Input: part model. Units: mm. Frame: model coordinates. Face numbers are marked on the shaded views. A direction names the side the tool comes from. Coordinates: 2 decimals unless noted, no trailing zeros. Loops run counter-clockwise (first coordinate to the right, second up) from the corner with the lowest first, then second, coordinate; pieces in that order, holes last. Notation, with made-up numbers: M -24,51 L 3,51 A24 cw 3,79 Z; hole C -26.5,7 d10. An arc over 180 degrees is marked long. Use a Markdown table: item, result. Add a question column.
1. Section A-A on z = -8.5. Output: boundary loops of the cut face in (x, y), then the cut area to 3 significant figures.
2. Pin query (flat end, axial travel): pin 1 (5 mm diameter, centred on x = 27, z = -25.5, fed in from -Y); pin 2 (4 mm diameter, centred on x = 39.5, z = -31.5, fed in from -Y); pin 3 (2.5 mm diameter, centred on x = 46.5, z = -15, fed in from -Y); pin 4 (4 mm diameter, centred on x = 30, y = -5, fed in from +Z) (1 decimal). Return the tip coordinate at first contact, or that it passes through.
3. Section C-C on z = -15. Output: boundary loops of the cut face in (x, y).
4. Draft query along Z for the marked faces 4, 5 and 6. Return one class per face: +Z half, -Z half, draft (parallel to the pull), parting line (faces both ways), or undercut.
5. Set-up query: the marked faces 1, 2 and 3. Return all of +Z, -Z, +X, -X, +Y, -Y with unobstructed straight access to the full face (end or side cutting, diameter ignored); none if empty.
6. Section D-D on x = 41. Output: boundary loops of the cut face in (y, z), then the cut area to 3 significant figures.
7. Line query: L1, parallel to Z at x = 19, y = 6.4; L2, parallel to X at y = 5.3, z = -32; L3, parallel to Y at x = 30, z = -23. Output: solid intervals per line, ascending. Write a range as [from, to].
```python
from build123d import *
from build123d.topology import SkipClean

# Parameters (mm, degrees)
SKETCH1_W            = 60
SKETCH1_H            = 42
BOSS_EXTRUDE1_DEPTH  = 8
SKETCH3_W            = 10
SKETCH3_H            = 42
BOSS_EXTRUDE5_DEPTH  = 6
SKETCH5_W            = 14
SKETCH5_H            = 42
BOSS_EXTRUDE6_DEPTH  = 11
SKETCH6_R            = 3.2
CUT_EXTRUDE1_DEPTH   = 75.565407529
FILLET1_R            = 7
FILLET2_R            = 5
FILLET3_R            = 5
BOSS_EXTRUDE7_DEPTH  = 42
SKETCH9_W            = 5
SKETCH9_H            = 42
BOSS_EXTRUDE8_DEPTH  = 6
SKETCH11_W           = 15
SKETCH11_H           = 42
CUT_EXTRUDE2_DEPTH   = 76.921011584
SKETCH12_W           = 30
SKETCH12_H           = 42
CUT_EXTRUDE3_DEPTH   = 6
SKETCH15_W           = 42
SKETCH15_H           = 8
BOSS_EXTRUDE9_DEPTH  = 5
SKETCH16_W           = 42
SKETCH16_H           = 8
BOSS_EXTRUDE10_DEPTH = 5
CUT_EXTRUDE7_START   = -17
CUT_EXTRUDE7_DEPTH   = 17
BOSS_EXTRUDE11_START = -5
SKETCH17_R           = 4.15
SKETCH17_R_2         = 2.2
BOSS_EXTRUDE11_DEPTH = 5
SKETCH18_W           = 2
SKETCH18_H           = 42
CUT_EXTRUDE8_DEPTH   = 67.392770772
CUT_EXTRUDE9_START   = -6
SKETCH19_R           = 3.2
CUT_EXTRUDE9_DEPTH   = 6
CUT_EXTRUDE10_DEPTH  = 6
SKETCH21_W           = 6.443242803
SKETCH21_H           = 1.161907564
SKETCH21_W_2         = 5.84761327
SKETCH21_H_2         = 1.16
SKETCH21_W_3         = 6.146169824
CUT_EXTRUDE11_DEPTH  = 6
CUT_EXTRUDE12_DEPTH  = 3
BOSS_EXTRUDE12_DEPTH = 6
BOSS_EXTRUDE13_DEPTH = 6


with BuildPart() as part:
    # Sketch1 → Boss-Extrude1 (new body)
    with BuildSketch(Plane(origin=(0, 0, 0), x_dir=(1, 0, 0), z_dir=(0, 1, 0))):
        with Locations((30, 21)):
            Rectangle(SKETCH1_W, SKETCH1_H)
    extrude(amount=BOSS_EXTRUDE1_DEPTH)

    # Sketch3 → Boss-Extrude5 (add)
    with BuildSketch(Plane(origin=(0, 8, 0), x_dir=(1, 0, 0), z_dir=(0, 1, 0))):
        with Locations((30, 21)):
            Rectangle(SKETCH3_W, SKETCH3_H)
    extrude(amount=BOSS_EXTRUDE5_DEPTH)

    # Sketch5 → Boss-Extrude6 (add)
    with BuildSketch(Plane.XZ):
        with Locations((30, -21)):
            Rectangle(SKETCH5_W, SKETCH5_H)
    extrude(amount=BOSS_EXTRUDE6_DEPTH)

    # Sketch6 → Cut-Extrude1 (cut, through all)
    with BuildSketch(Plane(origin=(0, 0, -42), x_dir=(-1, 0, 0), z_dir=(0, 0, -1))):
        with Locations((-30, -5)):
            Circle(SKETCH6_R)
    extrude(amount=-CUT_EXTRUDE1_DEPTH, mode=Mode.SUBTRACT)

    # Fillet1
    fillet1_edges = [part.edges().sort_by_distance(p)[0] for p in [
        (23, -11, -21),
        (37, -11, -21),
    ]]
    fillet(fillet1_edges, radius=FILLET1_R - 0.0001)  # a hair under: the kernel refuses the full size

    # Fillet2
    fillet2_edges = [part.edges().sort_by_distance(p)[0] for p in [
        (23, 0, -21),
    ]]
    fillet(fillet2_edges, radius=FILLET2_R)

    # Fillet3
    fillet3_edges = [part.edges().sort_by_distance(p)[0] for p in [
        (37, 0, -21),
    ]]
    fillet(fillet3_edges, radius=FILLET3_R)

    # Sketch8 → Boss-Extrude7 (add)
    with BuildSketch(Plane(origin=(0, 0, -42), x_dir=(-1, 0, 0), z_dir=(0, 0, -1))):
        with BuildLine():
            Line((-41.958260743, -1), (-42.958260743, 0))
            Line((-42.958260743, 0), (-41.958260743, 0))
            ThreePointArc((-41.958260743, 0), (-38.573244741, -1.320099639), (-36.9756521, -4.583333333))
            ThreePointArc((-36.9756521, -4.583333333), (-34.739022403, -9.151860505), (-30, -11))
            ThreePointArc((-30, -11), (-25.260977597, -9.151860505), (-23.0243479, -4.583333333))
            ThreePointArc((-23.0243479, -4.583333333), (-21.426755259, -1.320099639), (-18.041739257, 0))
            Line((-18.041739257, 0), (-16.803044796, 0))
            Line((-16.803044796, 0), (-18.041739257, -1))
            ThreePointArc((-18.041739257, -1), (-20.749752058, -2.056079711), (-22.027826171, -4.666666667))
            ThreePointArc((-22.027826171, -4.666666667), (-24.583974397, -9.887840578), (-30, -12))
            ThreePointArc((-30, -12), (-35.416025603, -9.887840578), (-37.972173829, -4.666666667))
            ThreePointArc((-37.972173829, -4.666666667), (-39.250247942, -2.056079711), (-41.958260743, -1))
        make_face()
    extrude(amount=-BOSS_EXTRUDE7_DEPTH)

    # Sketch9 → Boss-Extrude8 (add)
    with BuildSketch(Plane(origin=(0, 8, 0), x_dir=(1, 0, 0), z_dir=(0, 1, 0))):
        with Locations((42.5, 21)):
            Rectangle(SKETCH9_W, SKETCH9_H)
        with Locations((17.5, 21)):
            Rectangle(SKETCH9_W, SKETCH9_H)
    extrude(amount=BOSS_EXTRUDE8_DEPTH)

    # Sketch11 → Cut-Extrude2 (cut, through all)
    with BuildSketch(Plane(origin=(0, 8, 0), x_dir=(1, 0, 0), z_dir=(0, 1, 0))):
        with Locations((52.5, 21)):
            Rectangle(SKETCH11_W, SKETCH11_H)
        with Locations((7.5, 21)):
            Rectangle(SKETCH11_W, SKETCH11_H)
    extrude(amount=-CUT_EXTRUDE2_DEPTH, mode=Mode.SUBTRACT)

    # Sketch12 → Cut-Extrude3 (cut)
    with BuildSketch(Plane(origin=(0, 14, 0), x_dir=(1, 0, 0), z_dir=(0, 1, 0))):
        with Locations((30, 21)):
            Rectangle(SKETCH12_W, SKETCH12_H)
    extrude(amount=-CUT_EXTRUDE3_DEPTH, mode=Mode.SUBTRACT)

    # Sketch15 → Boss-Extrude9 (add)
    with BuildSketch(Plane.ZY.offset(-15)):
        with Locations((-21, 4)):
            Rectangle(SKETCH15_W, SKETCH15_H)
    extrude(amount=BOSS_EXTRUDE9_DEPTH)

    # Sketch16 → Boss-Extrude10 (add)
    with BuildSketch(Plane(origin=(45, 0, 0), x_dir=(0, 0, -1), z_dir=(1, 0, 0))):
        with Locations((21, 4)):
            Rectangle(SKETCH16_W, SKETCH16_H)
    extrude(amount=BOSS_EXTRUDE10_DEPTH)

    # Cut-Extrude7: read off the stored shape, not the designer's step
    # Cut-Extrude7 outline → Cut-Extrude7 (cut)
    with BuildSketch(Plane(origin=(0, 8, 0), x_dir=(1, 0, 0), z_dir=(0, 1, 0)).offset(CUT_EXTRUDE7_START)):
        with BuildLine():
            ThreePointArc((45, 33.105667219), (36.85, 32), (45, 30.894332781))
            Line((45, 30.894332781), (45, 33.105667219))
        make_face()
        with BuildLine():
            ThreePointArc((45, 11.105667219), (36.85, 10), (45, 8.894332781))
            Line((45, 8.894332781), (45, 11.105667219))
        make_face()
        with BuildLine():
            ThreePointArc((15, 8.894332781), (23.15, 10), (15, 11.105667219))
            Line((15, 11.105667219), (15, 8.894332781))
        make_face()
        with BuildLine():
            ThreePointArc((15, 30.894332781), (23.15, 32), (15, 33.105667219))
            Line((15, 33.105667219), (15, 30.894332781))
        make_face()
    extrude(amount=CUT_EXTRUDE7_DEPTH, mode=Mode.SUBTRACT)

    # Sketch17 → Boss-Extrude11 (add)
    # profile 1 of 4: a face of its own
    with BuildSketch(Plane(origin=(0, 8, 0), x_dir=(1, 0, 0), z_dir=(0, 1, 0)).offset(BOSS_EXTRUDE11_START)):
        with Locations((41, 32)):
            Circle(SKETCH17_R)
        with Locations(Location((41, 32, 0), (0, 0, 270))):
            Circle(SKETCH17_R_2, mode=Mode.SUBTRACT)
    # profile 2 of 4: a face of its own
    with BuildSketch(Plane(origin=(0, 8, 0), x_dir=(1, 0, 0), z_dir=(0, 1, 0)).offset(BOSS_EXTRUDE11_START)):
        with Locations((19, 10)):
            Circle(SKETCH17_R)
        with Locations(Location((19, 10, 0), (0, 0, 270))):
            Circle(SKETCH17_R_2, mode=Mode.SUBTRACT)
    # profile 3 of 4: a face of its own
    with BuildSketch(Plane(origin=(0, 8, 0), x_dir=(1, 0, 0), z_dir=(0, 1, 0)).offset(BOSS_EXTRUDE11_START)):
        with Locations((41, 10)):
            Circle(SKETCH17_R)
        with Locations(Location((41, 10, 0), (0, 0, 270))):
            Circle(SKETCH17_R_2, mode=Mode.SUBTRACT)
    # profile 4 of 4: a face of its own
    with BuildSketch(Plane(origin=(0, 8, 0), x_dir=(1, 0, 0), z_dir=(0, 1, 0)).offset(BOSS_EXTRUDE11_START)):
        with Locations((19, 32)):
            Circle(SKETCH17_R)
        with Locations(Location((19, 32, 0), (0, 0, 270))):
            Circle(SKETCH17_R_2, mode=Mode.SUBTRACT)
    extrude(amount=BOSS_EXTRUDE11_DEPTH)

    # Sketch18 → Cut-Extrude8 (cut, through all)
    with BuildSketch(Plane.XZ):
        with Locations((11, -21)):
            Rectangle(SKETCH18_W, SKETCH18_H)
        with Locations((49, -21)):
            Rectangle(SKETCH18_W, SKETCH18_H)
    extrude(amount=-CUT_EXTRUDE8_DEPTH, mode=Mode.SUBTRACT)

    # Sketch19 → Cut-Extrude9 (cut)
    with BuildSketch(Plane.XY.offset(CUT_EXTRUDE9_START)):
        with BuildLine():
            Line((48, 8), (48, 0))
            Line((48, 0), (42.958260743, 0))
            Line((42.958260743, 0), (41.958260743, -1))
            ThreePointArc((41.958260743, -1), (39.250247942, -2.056079711), (37.972173829, -4.666666667))
            ThreePointArc((37.972173829, -4.666666667), (30, -12), (22.027826171, -4.666666667))
            ThreePointArc((22.027826171, -4.666666667), (20.749752058, -2.056079711), (18.041739257, -1))
            Line((18.041739257, -1), (16.803044796, 0))
            Line((16.803044796, 0), (12, 0))
            Line((12, 0), (12, 8))
            Line((12, 8), (48, 8))
        make_face()
        with Locations(Location((30, -5, 0), (0, 0, 180))):
            Circle(SKETCH19_R, mode=Mode.SUBTRACT)
    extrude(amount=CUT_EXTRUDE9_DEPTH, mode=Mode.SUBTRACT)

    # Sketch20 → Cut-Extrude10 (cut)
    with BuildSketch(Plane(origin=(0, 0, -42), x_dir=(-1, 0, 0), z_dir=(0, 0, -1))):
        with BuildLine():
            Line((-16.803044796, 0), (-12, 0))
            Line((-12, 0), (-12, 8))
            Line((-12, 8), (-48, 8))
            Line((-48, 8), (-48, 0))
            Line((-48, 0), (-42.958260743, 0))
            Line((-42.958260743, 0), (-41.958260743, -1))
            ThreePointArc((-41.958260743, -1), (-39.250247942, -2.056079711), (-37.972173829, -4.666666667))
            ThreePointArc((-37.972173829, -4.666666667), (-30, -12), (-22.027826171, -4.666666667))
            ThreePointArc((-22.027826171, -4.666666667), (-20.749752058, -2.056079711), (-18.041739257, -1))
            Line((-18.041739257, -1), (-16.803044796, 0))
        make_face()
    extrude(amount=-CUT_EXTRUDE10_DEPTH, mode=Mode.SUBTRACT)

    # Sketch21 → Cut-Extrude11 (cut)
    with BuildSketch(Plane(origin=(0, 0, 0), x_dir=(-1, 0, 0), z_dir=(0, -1, 0))):
        with Locations((-18.806204769, 6.580953782)):
            Rectangle(SKETCH21_W, SKETCH21_H)
        with Locations((-19.104019536, 35.42)):
            Rectangle(SKETCH21_W_2, SKETCH21_H_2)
        with Locations((-41.045258741, 6.58)):
            Rectangle(SKETCH21_W_3, SKETCH21_H_2)
        with Locations((-41.045258741, 35.42)):
            Rectangle(SKETCH21_W_3, SKETCH21_H_2)
    extrude(amount=CUT_EXTRUDE11_DEPTH, mode=Mode.SUBTRACT)

    # Sketch22 → Cut-Extrude12 (cut, symmetric)
    with BuildSketch(Plane(origin=(0, 0, 0), x_dir=(-1, 0, 0), z_dir=(0, -1, 0))):
        Polygon((-36.85, 10), (-45, 10), (-45.05283361, 6), (-36.85, 6), align=None)
        Polygon((-45.05283361, 36), (-36.85, 36), (-36.85, 32), (-45, 32), align=None)
        Polygon((-14.94716639, 6), (-23.15, 6), (-23.15, 10), (-15, 10), align=None)
        Polygon((-15, 32), (-14.94716639, 36), (-23.15, 36), (-23.15, 32), align=None)
    extrude(amount=CUT_EXTRUDE12_DEPTH, both=True, mode=Mode.SUBTRACT)

    # Sketch24 → Boss-Extrude12 (add)
    with SkipClean():  # the faces are left unmerged after this step: merging them gives an invalid solid
        with BuildSketch(Plane(origin=(0, -3, 0), x_dir=(1, 0, 0), z_dir=(0, 1, 0))):
            with BuildLine():
                Line((22.027826171, 34.84), (22.026037012, 34.84))
                ThreePointArc((22.026037012, 34.84), (22.858792143, 33.527161812), (23.15, 32))
                Line((23.15, 32), (23.15, 36))
                Line((23.15, 36), (22.027826171, 36))
                Line((22.027826171, 36), (22.027826171, 34.84))
            make_face()
        extrude(amount=BOSS_EXTRUDE12_DEPTH)

    # Sketch25 → Boss-Extrude13 (add)
    with SkipClean():  # the faces are left unmerged after this step: merging them gives an invalid solid
        with BuildSketch(Plane(origin=(0, -3, 0), x_dir=(1, 0, 0), z_dir=(0, 1, 0))):
            with BuildLine():
                Line((37.973962988, 34.84), (37.972173829, 34.84))
                Line((37.972173829, 34.84), (37.972173829, 36))
                Line((37.972173829, 36), (36.85, 36))
                Line((36.85, 36), (36.85, 32))
                ThreePointArc((36.85, 32), (37.141207857, 33.527161812), (37.973962988, 34.84))
            make_face()
            with BuildLine():
                Line((36.85, 10), (36.85, 6))
                Line((36.85, 6), (37.972173829, 6))
                Line((37.972173829, 6), (37.972173829, 7.16))
                Line((37.972173829, 7.16), (37.973962988, 7.16))
                ThreePointArc((37.973962988, 7.16), (37.141207857, 8.472838188), (36.85, 10))
            make_face()
            with BuildLine():
                Line((22.027826171, 7.161907564), (22.027826171, 6))
                Line((22.027826171, 6), (23.15, 6))
                Line((23.15, 6), (23.15, 10))
                ThreePointArc((23.15, 10), (22.859273158, 8.474054164), (22.027826171, 7.161907564))
            make_face()
        extrude(amount=BOSS_EXTRUDE13_DEPTH)


solid = part.part
```
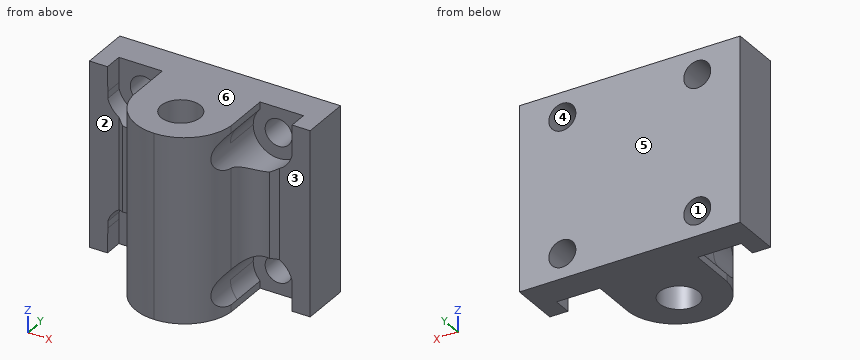
Answers below:
| question | item | result |
|---|---|---|
| 1 | outline | M 12,0 L 14.98,0 L 14.98,3 L 17.39,3 L 17.39,8 L 12,8 Z; M 20.61,3 L 22.87,3 L 22.87,-7.63 A8 ccw 37.13,-7.63 L 37.13,3 L 39.39,3 L 39.39,8 L 20.61,8 Z; M 42.61,3 L 45.02,3 L 45.02,0 L 48,0 L 48,8 L 42.61,8 Z; hole C 30,-5 d6.4 |
| 1 | area | 330 mm² |
| 2 | pin 1 | stops at y = -11.98 |
| 2 | pin 2 | stops at y = 3 |
| 2 | pin 3 | stops at y = 0 |
| 2 | pin 4 | passes through |
| 3 | outline | M 12,0 L 16.8,0 L 18.04,-1 A4 cw 22.03,-4.67 A8 ccw 37.97,-4.67 A4 cw 41.96,-1 L 42.96,0 L 48,0 L 48,8 L 12,8 Z; hole C 30,-5 d6.4 |
| 4 | face 4 | undercut |
| 4 | face 5 | draft |
| 4 | face 6 | +Z half |
| 5 | face 1 | +Y, -Y |
| 5 | face 2 | +Z, -Z, -X, -Y |
| 5 | face 3 | +Z, -Z, +X, -Y |
| 6 | outline | M -1.12,-27.85 L 3,-27.85 L 3,-29.8 L 8,-29.8 L 8,-12.2 L 3,-12.2 L 3,-14.15 L -1.12,-14.15 Z; M 3,-36 L 8,-36 L 8,-34.2 L 3,-34.2 Z; M 3,-7.8 L 8,-7.8 L 8,-6 L 3,-6 Z |
| 6 | area | 162 mm² |
| 7 | L1 | z = [-36, -34.2], [-29.8, -12.2], [-7.8, -6] |
| 7 | L2 | x = [12, 16.8], [21.2, 38.8], [43.2, 48] |
| 7 | L3 | y = [-12, -8.2], [-1.8, 8] |
